Here's how the part is built. I have some questions about the finished solid (model axes, mm). Face numbers are marked on the shaded views. A direction names the side the tool comes from. Coordinates: 2 decimals unless noted, no trailing zeros. Loops run counter-clockwise (first coordinate to the right, second up) from the corner with the lowest first, then second, coordinate; pieces in that order, holes last. Notation, with made-up numbers: (80.25, -20) - (107.25, -20) arc R32 cw to (107.25, 17) - close; hole circle Ø5 at (39, 0). An arc over 180 degrees is marked (long way). Use a Markdown table: item, result.
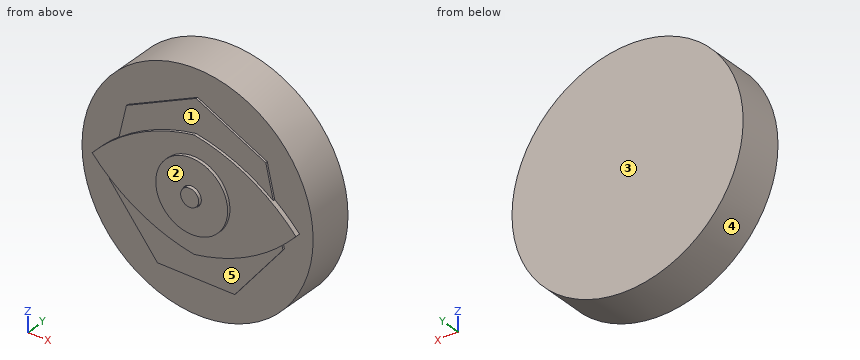
```python
from build123d import *

# Parameters (mm, degrees)
F0_R     = 76.270958
F1_DEPTH = 29.972
F3_DEPTH = 33.02
F5_DEPTH = 31.242
F6_R     = 23.721121
F6_R_2   = 6.37486
F7_DEPTH = 35.052
F8_R     = 5.929378
F9_DEPTH = 36.83


with BuildPart() as f1:
    # F0 (on Front) → F1 (new body)
    with BuildSketch(Plane.XZ):
        Circle(F0_R)
    extrude(amount=F1_DEPTH)

    # F2 (on Front) → F3 (join)
    with BuildSketch(Plane.XZ):
        with BuildLine():
            ThreePointArc((67.254432, 0), (36.779267, 24.243834), (0, 37.041672))
            ThreePointArc((0, 37.041672), (-36.779267, 24.243834), (-67.254432, 0))
            ThreePointArc((-67.254432, 0), (-36.779267, -24.243834), (0, -37.041672))
            ThreePointArc((0, -37.041672), (36.779267, -24.243834), (67.254432, 0))
        make_face()
    extrude(amount=F3_DEPTH)

    # F4 (on Front) → F5 (join)
    with BuildSketch(Plane.XZ):
        Polygon((-25.51971, -52.992225), (25.51971, -52.992225), (57.342269, -13.087999), (45.984929, 36.671757), (0, 58.816932), (-45.984929, 36.671757), (-57.342269, -13.087999), align=None)
    extrude(amount=F5_DEPTH)

    # F6 (on Front) → F7 (join)
    with BuildSketch(Plane.XZ):
        Circle(F6_R)
        Circle(F6_R_2, mode=Mode.SUBTRACT)
    extrude(amount=F7_DEPTH)

    # F8 (on Front) → F9 (join)
    with BuildSketch(Plane.XZ):
        Circle(F8_R)
    extrude(amount=F9_DEPTH)


solid = f1.part
```
Q1. I want a section at B-B, the plane x = 64.5. Write out the boundary of the cut face in (y, z).
Check values:
| item | result |
|---|---|
| outline | (-33.02, -2.97) - (-29.97, -2.97) - (-29.97, -40.71) - (0, -40.71) - (0, 40.71) - (-29.97, 40.71) - (-29.97, 2.97) - (-33.02, 2.97) - close |
Q2. Which directions (+Z, -Z, +X, -X, +Y, -Y) give clear straight access to the entire face, cutting with the end or side of a thin tool? Please do the marked faces 1, 2, 3, 4 and 5.
Check values:
| item | result |
|---|---|
| face 1 | +Z, -Y |
| face 2 | -Y |
| face 3 | +Z, -Z, +X, -X, +Y |
| face 4 | +Y, -Y |
| face 5 | -Z, -Y |
Q3. Please list where these lines run through material, in increasing order: L1, parallel to X at y = -34.45, z = 0; L2, parallel to Y at x = -41.5, z = -23. Write a range as from..to.
Check values:
| item | result |
|---|---|
| L1 | -23.72..-6.37, -5.93..5.93, 6.37..23.72 |
| L2 | -31.24..0 |
Q4. I want a section at A-A, the plane z = 19. Write out the boundary of the cut face in (x, y), then the cut area to 3 significant figures.
Check values:
| item | result |
|---|---|
| outline | (-73.87, -29.97) - (-50.02, -29.97) - (-50.02, -31.24) - (-45.39, -31.24) - (-45.39, -33.02) - (-14.2, -33.02) - (-14.2, -35.05) - (14.2, -35.05) - (14.2, -33.02) - (45.39, -33.02) - (45.39, -31.24) - (50.02, -31.24) - (50.02, -29.97) - (73.87, -29.97) - (73.87, 0) - (-73.87, 0) - close |
| area | 4,770 mm^2 |
Q5. I want a section at D-D, the plane z = -44. Write out the boundary of the cut face in (x, y).
Check values:
| item | result |
|---|---|
| outline | (-62.3, -29.97) - (-32.69, -29.97) - (-32.69, -31.24) - (32.69, -31.24) - (32.69, -29.97) - (62.3, -29.97) - (62.3, 0) - (-62.3, 0) - close |
Q6. Will these pins go through, and if not, where does the flat tip stop? P1, Ø14, axis at x = -11.5, z = 6.5, coming from the -Y side; P2, Ø1.5, axis at y = -19, z = -47.5, coming from the +X side; P3, Ø12, axis at x = 56.5, y = -10.5, coming from the -Z side.
Check values:
| item | result |
|---|---|
| P1 | y = -35.05 |
| P2 | x = 60.26 |
| P3 | z = -57.16 |
Q7. I want a section at C-C, the plane y = -8. Write out the boundary of the cut face in (x, z).
Check values:
| item | result |
|---|---|
| outline | circle Ø152.54 at (0, 0) |
